```python
from build123d import *

# Parameters (mm, degrees)
F1_DEPTH      = 400
F1_DEPTH_BACK = 400


with BuildPart() as f1:
    # F0 (on Right) → F1 (new body, two sides)
    with BuildSketch(Plane.YZ) as f1_sk:
        Polygon((-957, -175), (1092, -175), (1225, -45), (1225, 175), (-962.085426, 175), (-1225, 42), align=None)
    extrude(amount=F1_DEPTH)
    extrude(f1_sk.sketch, amount=-F1_DEPTH_BACK)


solid = f1.part
```
For this review, take the finished solid that the model builds, in its own axes (mm). Give positions to 0.01 mm unless a question says otherwise; leave off trailing zeros. Order: outer loops, then holes, each group sorted by start corner. A loop starts at its lowest first (then second) coordinate and runs counter-clockwise, first axis right, second up.
1) Insertion check: pin 1 (4 mm diameter, centred on x = -23.5, y = -974, fed in from +Z); pin 2 (10 mm diameter, centred on x = 11.5, z = -73, fed in from +Y); pin 3 (4 mm diameter, centred on x = 126.5, z = -90.5, fed in from -Y). Each pin has a flat end and moves straight along its axis. Give the tip position at first contact, or say it passes through.
2) Take a section at C-C (z = 131). Give the boundary of the cut face in (x, y), then the cut area to 3 significant figures.
3) Wall thickness on line 1 (Y direction, x = -215.5, z = 76); line 2 (Y direction, x = -166.5, z = 111): over which ranges is each line inside the solid? List them lowest first.
4) Take a section at A-A (x = -241.5). Give the boundary of the cut face in (y, z).
5) Take a section at B-B (z = 10). Give the boundary of the cut face in (x, y).
Derived:
1. pin 1: stops at z = 169.98
1. pin 2: stops at y = 1201.47
1. pin 3: stops at y = -1063.83
2. outline: (-400, -1049.06) - (400, -1049.06) - (400, 1225) - (-400, 1225) - close
2. area: 1,820,000 mm2
3. line 1: y = -1157.79 to 1225
3. line 2: y = -1088.6 to 1225
4. outline: (-1225, 42) - (-957, -175) - (1092, -175) - (1225, -45) - (1225, 175) - (-962.09, 175) - close
5. outline: (-400, -1185.48) - (400, -1185.48) - (400, 1225) - (-400, 1225) - close
